Geometry: final body of the model. Coordinates: model frame, mm. Face numbers are marked on the shaded views. A direction names the side the tool comes from. Give positions to 0.01 mm unless a question says otherwise; leave off trailing zeros. Write each loop counter-clockwise with the first axis right and the second up, starting at its lowest first coordinate (ties: lowest second). Pieces come first, ordered by that corner, then holes.
Q1. Reachability of the marked faces 1 and 2 from +Z, -Z, +X, -X, +Y, -Y: full face, straight path, thin tool, end or side. Return the list, or none.
Q2. Cut plane B-B on y = 12. Return the cut outline in (x, z), plus the area to 3 significant figures.
Q3. Draft query along Z for the marked faces 3, 4, 5 and 6. Return one class per face: pulls with the +Z half, pulls with the -Z half, needs draft (parallel to the pull), parting line crosses it, or undercut.
Q4. Cut plane C-C on x = 10.5. Return the cut outline in (y, z).
Q5. Line query: L1, parallel to Z at x = -16, y = 0; L2, parallel to X at y = 1.5, z = 10.75; L3, parallel to X at y = 0, z = 9.75. Output: solid intervals per line, ascending.
Q6. Cut plane A-A on z = 22. Return the cut outline in (x, y), plus the area to 3 significant figures.
Q7. Cut plane D-D on z = 13.25. Return the cut outline in (x, y).
Q8. Pin query (flat end, axial travel): pin 1 (10 mm diameter, centred on y = 10, z = 4, fed in from +X) (3 decimals); pin 2 (2 mm diameter, centred on x = 1, z = 18, fed in from -Y); pin 3 (4 mm diameter, centred on y = -2, z = 5, fed in from +X). Return the tip coordinate at first contact, or that it passes through.
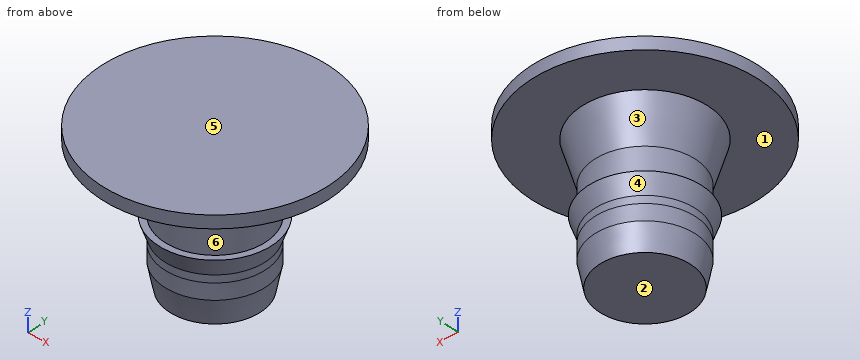
```python
from build123d import *


with BuildPart() as f1:
    # F0 (on Front) → F1 (revolve)
    with BuildSketch(Plane.XZ):
        Polygon((-8.001124, 7.66683), (-8.001124, 6.5), (-8, 4), (-7.2, 0), (0, 0), (0, 23.5), (-18.001124, 23.5), (-18.001124, 21.5), (-10.001124, 21.5), (-8.001124, 21.5), (-8.001124, 14.782405), (-8.001124, 10.5), align=None)
        Polygon((-9.001124, 10.5), (-8.001124, 7.66683), (-8.001124, 10.5), align=None)
        Polygon((-10.001124, 21.5), (-8.001124, 14.782405), (-8.001124, 21.5), align=None)
    revolve(axis=Axis((0, 0, 11.75), (0, 0, -1)))


solid = f1.part
```
Data:
1. face 1: -Z
1. face 2: -Z, +X, -X, +Y, -Y
2. outline: (-13.42, 21.5) - (13.42, 21.5) - (13.42, 23.5) - (-13.42, 23.5) - close
2. area: 53.7 mm2
3. face 3: undercut
3. face 4: pulls with the -Z half
3. face 5: pulls with the +Z half
3. face 6: undercut
4. outline: (-14.62, 21.5) - (14.62, 21.5) - (14.62, 23.5) - (-14.62, 23.5) - close
5. L1: z = 21.5 to 23.5
5. L2: x = -7.86 to 7.86
5. L3: x = -8.74 to 8.74
6. outline: circle Ø36 at (0, 0)
6. area: 1,020 mm2
7. outline: circle Ø16 at (0, 0)
8. pin 1: stops at x = 6.245
8. pin 2: stops at y = -9.22
8. pin 3: stops at x = 8
